from build123d import *


with BuildPart() as part:
    # Esquisse1 → Révolution1 (revolve)
    with BuildSketch(Plane(origin=(0, 0, 0), x_dir=(0, 0, -1), z_dir=(1, 0, 0)), mode=Mode.PRIVATE) as r_volution1_sk:
        with BuildLine():
            Line((3.7367497, 7.3), (4.5, 7.1))
            Line((4.5, 7.1), (4.5, 6.75))
            Line((4.5, 6.75), (4.1, 6.5))
            Line((4.1, 6.5), (3.5, 6))
            Line((3.5, 6), (1.1, 7))
            Line((1.1, 7), (0.5, 6.25))
            Line((0.5, 6.25), (0.2, 6.5))
            Line((0.2, 6.5), (0.5, 7.25))
            Line((0.5, 7.25), (0, 8))
            Line((0, 8), (0, 10.5))
            Line((0, 10.5), (0.5, 11))
            Line((0.5, 11), (4.5, 11))
            Line((4.5, 11), (5, 10.5))
            Line((5, 10.5), (5, 10))
            Line((5, 10), (1, 10))
            Line((1, 10), (1, 8.6))
            Line((1, 8.6), (1.883484861, 8.05))
            ThreePointArc((1.883484861, 8.05), (3.175136454, 8.576969601), (3.7367497, 7.3))
        make_face()
    revolve(r_volution1_sk.sketch.rotate(Axis((0, 0, 0), (0, 0, -1)), 90), axis=Axis((0, 0, 0), (0, 0, -1)))


solid = part.part
Can you work these out from the model? Positions are in its coordinate system, mm. A direction names the side the tool comes from. Round coordinates to 2 decimals unless told otherwise and drop trailing zeros. Use a Markdown table: item, result.
Item 1: For pin 1 Ø12 at (x, y) = (-4.5, 4.5) entering from -Z; pin 2 Ø1 at (x, z) = (-7, -4.5) entering from -Y; pin 3 Ø1.5 at (x, z) = (-7.5, -4) entering from -Y; pin 4 Ø4.5 at (x, y) = (1, -3.5) entering from -Z, each with a flat end and sliding along its axis, tell me the tip position at first contact or that it passes through.
Found:
| item | result |
|---|---|
| pin 1 | stops at z = -5 |
| pin 2 | stops at y = -8.87 |
| pin 3 | stops at y = -8.69 |
| pin 4 | passes through |
Item 2: If I drill on line 1 along Y through (x, z) = (0, -3); line 2 along Y through (x, z) = (-0.5, -1.5); line 3 along X through (y, z) = (-3.5, -1.55), over which ranges is the centre line in solid material (lowest first)? Write a range as [from, to].
Found:
| item | result |
|---|---|
| line 1 | y = [-11, -10], [-8.63, -6.21], [6.21, 8.63], [10, 11] |
| line 2 | y = [-10.99, -9.99], [-8.27, -6.82], [6.82, 8.27], [9.99, 10.99] |
| line 3 | x = [-10.43, -9.37], [-7.48, -5.84], [5.84, 7.48], [9.37, 10.43] |
Item 3: Which directions (+Z, -Z, +X, -X, +Y, -Y) give clear straight access to the entire face, cutting with the end or side of a thin tool? Please do faces 4 (the face through (2, 8, 0)), 5 (the face through (5.783, -1.821, -3.35)).
Found:
| item | result |
|---|---|
| face 4 | +Z, +X, -X, +Y, -Y |
| face 5 | none |
Item 4: We'd pull the mould along X, two halves only. Please class faces 1 (the face through (-2.38, 10.74, -2.53)), 2 (the face through (5, 9, -5)), 3 (the face through (-10, 0, -3)): released by +X, released by -X, zero draft, split by the parting line, or undercut.
Found:
| item | result |
|---|---|
| face 1 | split by the parting line |
| face 2 | zero draft |
| face 3 | undercut |
